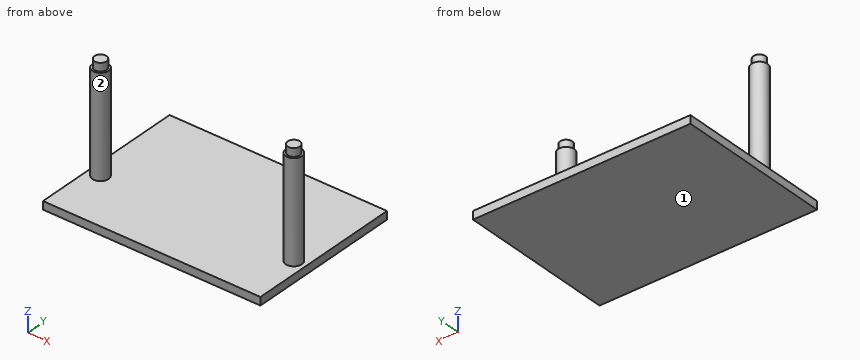
```python
from build123d import *

# Parameters (mm, degrees)
SKETCH_W     = 54
SKETCH_H     = 39
PAD_DEPTH    = 2
SKETCH001_R  = 2
PAD001_DEPTH = 25
SKETCH002_R  = 1.5
PAD002_DEPTH = 2
SKETCH003_R  = 1.5
PAD003_DEPTH = 2


with BuildPart() as part:
    # Sketch → Pad (new body)
    with BuildSketch(Plane.XY):
        with Locations((27, 19.5)):
            Rectangle(SKETCH_W, SKETCH_H)
    extrude(amount=PAD_DEPTH)

    # Sketch001 (on Face6 of Pad) → Pad001 (join)
    with BuildSketch(Plane.XY.offset(2)):
        with Locations((3, 14)):
            Circle(SKETCH001_R)
        with Locations((51, 14)):
            Circle(SKETCH001_R)
    extrude(amount=PAD001_DEPTH)

    # Sketch002 (on Face9 of Pad001) → Pad002 (join)
    with BuildSketch(Plane.XY.offset(27)):
        with Locations((51, 14)):
            Circle(SKETCH002_R)
    extrude(amount=PAD002_DEPTH)

    # Sketch003 (on Face9 of Pad002) → Pad003 (join)
    with BuildSketch(Plane.XY.offset(27)):
        with Locations((3, 14)):
            Circle(SKETCH003_R)
    extrude(amount=PAD003_DEPTH)


solid = part.part
```
Can you work these out from the model? Positions are in its coordinate system, mm. Face numbers are marked on the shaded views. Coordinates: 2 decimals unless noted, no trailing zeros. Loops run counter-clockwise (first coordinate to the right, second up) from the corner with the lowest first, then second, coordinate; pieces in that order, holes last.
1) Imagine slicing it at B-B on z = 5.75. List the corners of the cut face in (x, y) for me, plus the area to 3 significant figures.
2) Imagine slicing it at C-C on y = 14. List the corners of the cut face in (x, z) for me, plus the area to 3 significant figures.
3) Thinking about a two-plate mould opening in X: for the marked faces 1 and 2, which applies, pulls with the +X half, pulls with the -X half, needs draft (parallel to the pull), parting line crosses it, or undercut?
4) Imagine slicing it at D-D on x = 12. List the corners of the cut face in (y, z) for me, plus the area to 3 significant figures.
5) I need wall thicknesses on probe 1 along Z at (x, y) = (38.5, 2.5); probe 2 along Y at (x, z) = (4.5, 12). Which ranges of each line are inside material? Lowest first, please.
6) Imagine slicing it at A-A on x = 51. List the corners of the cut face in (y, z) for me.
7) For pin 1 (2 mm diameter, centred on y = 18, z = 23.5, fed in from +X); pin 2 (19.5 mm diameter, centred on x = 37, y = 26.5, fed in from +Z); pin 3 (10 mm diameter, centred on y = 19, z = 14, fed in from -X), each with a flat end and sliding along its axis, tell me the tip position at first contact or that it passes through.
Completed:
1. outline: circle Ø4 at (3, 14); circle Ø4 at (51, 14)
1. area: 25.1 mm2
2. outline: (0, 0) - (54, 0) - (54, 2) - (53, 2) - (53, 27) - (52.5, 27) - (52.5, 29) - (49.5, 29) - (49.5, 27) - (49, 27) - (49, 2) - (5, 2) - (5, 27) - (4.5, 27) - (4.5, 29) - (1.5, 29) - (1.5, 27) - (1, 27) - (1, 2) - (0, 2) - close
2. area: 320 mm2
3. face 1: needs draft
3. face 2: undercut
4. outline: (0, 0) - (39, 0) - (39, 2) - (0, 2) - close
4. area: 78.0 mm2
5. probe 1: z = 0 to 2
5. probe 2: y = 12.68 to 15.32
6. outline: (0, 0) - (39, 0) - (39, 2) - (16, 2) - (16, 27) - (15.5, 27) - (15.5, 29) - (12.5, 29) - (12.5, 27) - (12, 27) - (12, 2) - (0, 2) - close
7. pin 1: passes through
7. pin 2: stops at z = 2
7. pin 3: stops at x = 1
